Part print with two shaded views. Sizes in mm from the minimum x, y, z corner. A direction names the side the tool comes from. Coordinates: 2 decimals unless noted, no trailing zeros. Order: outer loops, then holes, each group sorted by start corner. A loop starts at its lowest first (then second) coordinate and runs counter-clockwise, first axis right, second up.
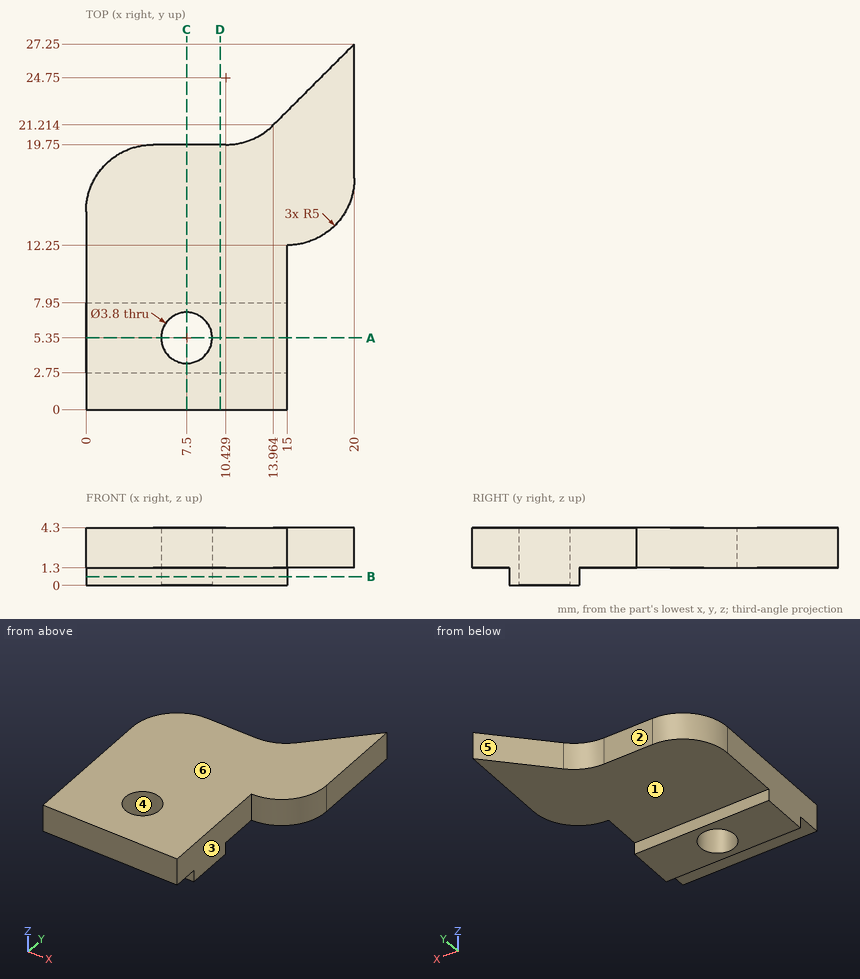
Q1. Cut at B-B on z = 0.65. Write the cut outline in (x, y).
Results list:
outline: (0, 2.75) - (15, 2.75) - (15, 7.95) - (0, 7.95) - close; hole circle Ø3.8 at (7.5, 5.35)
Q2. Cut at A-A on y = 5.35. Write the cut outline in (x, z).
Results list:
outline: (0, 0) - (5.6, 0) - (5.6, 4.3) - (0, 4.3) - close; (9.4, 0) - (15, 0) - (15, 4.3) - (9.4, 4.3) - close
Q3. Wall check: line 1 along Y through (x, z) = (7.5, 2.6); line 2 along Z through (x, y) = (1.5, 16.5); line 3 along X through (y, z) = (8.5, 4). Give the ranges that are in metal, low to high.
Results list:
line 1: y = 0 to 3.45, 7.25 to 19.75
line 2: z = 1.3 to 4.3
line 3: x = 0 to 15
Q4. Cut at C-C on x = 7.5. Write the cut outline in (y, z).
Results list:
outline: (0, 1.3) - (2.75, 1.3) - (2.75, 0) - (3.45, 0) - (3.45, 4.3) - (0, 4.3) - close; (7.25, 0) - (7.95, 0) - (7.95, 1.3) - (19.75, 1.3) - (19.75, 4.3) - (7.25, 4.3) - close
Q5. Which spindle directions (+Z, -Z, +X, -X, +Y, -Y) get a long thin tool onto all of the face, cutting with end or side? Do the marked faces 1, 2 and 3. Say none if no direction does.
Results list:
face 1: -Z, +X, -X, +Y
face 2: +Z, -Z, -X, +Y
face 3: +Z, -Z, +X, -Y
Q6. Cut at D-D on x = 10. Write the cut outline in (y, z).
Results list:
outline: (0, 1.3) - (2.75, 1.3) - (2.75, 0) - (7.95, 0) - (7.95, 1.3) - (19.75, 1.3) - (19.75, 4.3) - (0, 4.3) - close
Q7. Pin check, flat tips, straight feed: pin 1 Ø6 at (x, y) = (9, 14) entering from -Z; pin 2 Ø1.3 at (y, z) = (5, 3) entering from +X; pin 3 Ø6 at (x, y) = (7.5, 5.35) entering from -Z; pin 4 Ø1.4 at (x, z) = (5.5, 0.5) entering from -Y. Stop position of each tip, or through.
Results list:
pin 1: stops at z = 1.3
pin 2: stops at x = 15
pin 3: stops at z = 0
pin 4: stops at y = 2.75
Q8. Mould opens along Y. For the marked faces 4, 5 and 6 say: pulls with the +Y half, pulls with the -Y half, needs draft (parallel to the pull), parting line crosses it, or undercut.
Results list:
face 4: undercut
face 5: pulls with the +Y half
face 6: needs draft
